The figure shows three views and two pictorial views of one solid part (mm, origin at its lowest corner). Answer the questions. A direction names the side the tool comes from. Coordinates: 2 decimals unless noted, no trailing zeros. Write each loop counter-clockwise with the first axis right and the second up, starting at its lowest first coordinate (ties: lowest second). Pieces come first, ordered by that corner, then holes. Notation, with made-up numbers: M 73.25,12.5 L 115.25,12.5 A18 ccw 115.25,27.5 Z; hole C -17,19.25 d5. An arc over 180 degrees is marked long. Use CSV: the item, a comma, the result in double quotes.
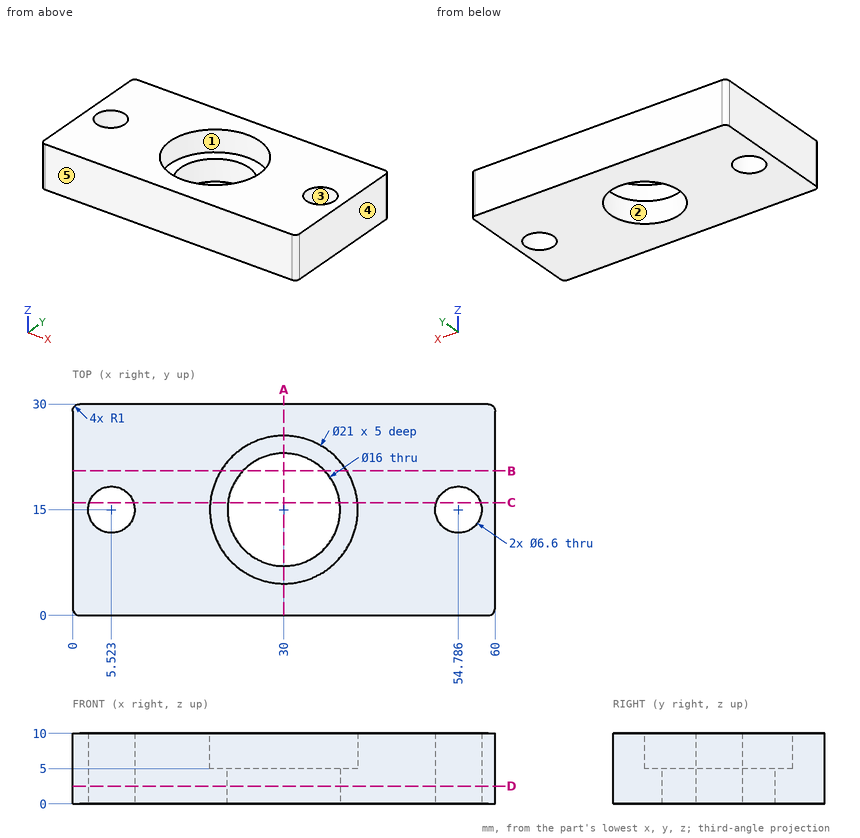
Item 1: The part is cut by section A-A (x = 30). Write down the section's boundary in (y, z).
Answer:
outline,"M 0,0 L 7,0 L 7,5 L 4.5,5 L 4.5,10 L 0,10 Z; M 23,0 L 30,0 L 30,10 L 25.5,10 L 25.5,5 L 23,5 Z"
Item 2: The part is cut by section C-C (y = 16). Write down the section's boundary in (x, z).
Answer:
outline,"M 0,0 L 2.38,0 L 2.38,10 L 0,10 Z; M 8.67,0 L 22.06,0 L 22.06,5 L 19.55,5 L 19.55,10 L 8.67,10 Z; M 37.94,0 L 51.64,0 L 51.64,10 L 40.45,10 L 40.45,5 L 37.94,5 Z; M 57.93,0 L 60,0 L 60,10 L 57.93,10 Z"
Item 3: The part is cut by section B-B (y = 20.5). Write down the section's boundary in (x, z).
Answer:
outline,"M 0,0 L 24.19,0 L 24.19,5 L 21.06,5 L 21.06,10 L 0,10 Z; M 35.81,0 L 60,0 L 60,10 L 38.94,10 L 38.94,5 L 35.81,5 Z"
Item 4: The part is cut by section D-D (z = 2.5). Write down the section's boundary in (x, y), then the cut area to 3 significant figures.
Answer:
outline,"M 0,1 A1 ccw 1,0 L 59,0 A1 ccw 60,1 L 60,29 A1 ccw 59,30 L 1,30 A1 ccw 0,29 Z; hole C 5.52,15 d6.6; hole C 30,15 d16; hole C 54.79,15 d6.6"
area,"1,530 mm2"
Item 5: Consider probe 1 along Y at (x, z) = (30, 6.5); probe 2 along Y at (x, z) = (30, 2.8); probe 3 along X at (y, z) = (17.25, 9) (1 decimal). Determine where each line is inside the solid, lowest interval first.
Answer:
probe 1,"y = 0 to 4.5, 25.5 to 30"
probe 2,"y = 0 to 7, 23 to 30"
probe 3,"x = 0 to 3.1, 7.9 to 19.7, 40.3 to 52.4, 57.2 to 60"
Item 6: A tool of negligible diameter and unlimited length cuts with its end or side. For the marked faces 1 and 2, from which of +Z, -Z, +X, -X, +Y, -Y can it reach the whole face along a straight path? Write none if from no direction.
Answer:
face 1,"+Z"
face 2,"+Z, -Z"
Item 7: For a pull along X with two mould halves and no side action, classify the marked faces 3, 4 and 5 as released by +X, released by -X, zero draft, split by the parting line, or undercut.
Answer:
face 3,"undercut"
face 4,"released by +X"
face 5,"zero draft"
